Can you work these out from the model? Positions are in its coordinate system, mm. Face numbers are marked on the shaded views. Give positions to 0.01 mm unless a question says otherwise; leave off trailing zeros. Order: outer loops, then holes, each group sorted by start corner. A loop starts at its lowest first (then second) coordinate and runs counter-clockwise, first axis right, second up. Notation, with made-up numbers: M 15.25,74.5 L 23.25,74.5 A7 ccw 23.25,87.5 Z; hole C -3.75,-38.75 d5. An arc over 180 degrees is marked long. Write each question's results on one line, items separated by ' | '.
from build123d import *

# Parameters (mm, degrees)
F0_R     = 6.35
F1_DEPTH = 25.4


with BuildPart() as f1:
    # F0 (on Front) → F1 (new body)
    with BuildSketch(Plane.XZ):
        with BuildLine():
            Line((0, -3.317883), (0, 15.07361))
            Line((0, 15.07361), (-15.875, 15.07361))
            Line((-15.875, 15.07361), (-50.8, -3.97639))
            Line((-50.8, -3.97639), (-50.8, -48.42639))
            Line((-50.8, -48.42639), (0, -48.42639))
            Line((0, -48.42639), (0, -30.034896))
            ThreePointArc((0, -30.034896), (-13.358506, -16.67639), (0, -3.317883))
        make_face()
        with Locations((-31.75, -29.37639)):
            Circle(F0_R, mode=Mode.SUBTRACT)
        with BuildLine():
            Line((15.875, 15.07361), (0, 15.07361))
            Line((0, 15.07361), (0, -3.317883))
            ThreePointArc((0, -3.317883), (13.358506, -16.67639), (0, -30.034896))
            Line((0, -30.034896), (0, -48.42639))
            Line((0, -48.42639), (50.8, -48.42639))
            Line((50.8, -48.42639), (50.8, -3.97639))
            Line((50.8, -3.97639), (15.875, 15.07361))
        make_face()
        with Locations((31.75, -29.37639)):
            Circle(F0_R, mode=Mode.SUBTRACT)
    extrude(amount=F1_DEPTH)


solid = f1.part
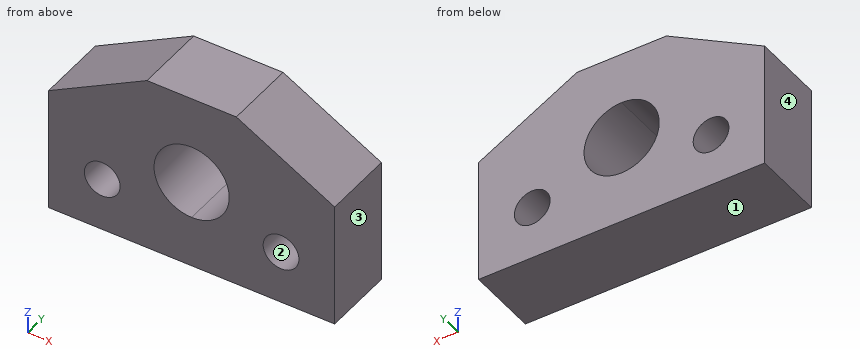
(1) Imagine slicing it at C-C, the plane z = -16. Write out the boundary of the cut face in (x, y), plus the area to 3 significant figures.
Data:
outline: M -50.8,-25.4 L -13.34,-25.4 L -13.34,0 L -50.8,0 Z; M 13.34,-25.4 L 50.8,-25.4 L 50.8,0 L 13.34,0 Z | area: 1,900 mm2
(2) Imagine slicing it at A-A, the plane x = -35. Write out the boundary of the cut face in (y, z), plus the area to 3 significant figures.
Data:
outline: M -25.4,-48.43 L 0,-48.43 L 0,-34.83 L -25.4,-34.83 Z; M -25.4,-23.92 L 0,-23.92 L 0,4.64 L -25.4,4.64 Z | area: 1,070 mm2
(3) Imagine slicing it at D-D, the plane z = -0.5. Write out the boundary of the cut face in (x, y).
Data:
outline: M -44.43,-25.4 L 44.43,-25.4 L 44.43,0 L -44.43,0 Z
(4) Will these pins go through, and if not, where does the flat tip stop? P1, Ø3, axis at y = -7, z = 3, coming from the -X side; P2, Ø16.5, axis at x = 31.75, z = -29.38, coming from the +Y side; P3, Ø10, axis at x = -31, y = -14, coming from the +Z side.
Data:
P1: stops at x = -40.76 | P2: stops at y = 0 | P3: stops at z = 9.55
(5) We'd pull the mould along X, two halves only. Please class the marked faces 1, 2, 3 and 4: +X half, -X half, draft (parallel to the pull), parting line (faces both ways), or undercut.
Data:
face 1: draft | face 2: undercut | face 3: +X half | face 4: -X half
(6) I need wall thicknesses on L1, parallel to Z at x = 31.75, y = -19.75; L2, parallel to X at y = -4.5, z = -8.5; L3, parallel to Z at x = -7, y = -13.25. Which ranges of each line are inside material? Lowest first, please. Write a range as from..to.
Data:
L1: z = -48.43..-35.73, -23.03..6.41 | L2: x = -50.8..-10.56, 10.56..50.8 | L3: z = -48.43..-28.05, -5.3..15.07
(7) Imagine slicing it at B-B, the plane y = -14. Count the separate pieces of the cut face and the enclosed holes in it, plus the area to 3 significant figures.
Data:
separate pieces: 1 | enclosed holes: 3 | area: 4,970 mm2
